Can you work these out from the model? Positions are in its coordinate system, mm. Give positions to 0.01 mm unless a question says otherwise; leave off trailing zeros. Order: outer loops, then holes, each group sorted by start corner. A loop starts at its lowest first (then second) coordinate and runs counter-clockwise, first axis right, second up. Notation, with made-up numbers: (15.25, 78.5) - (61.25, 78.5) arc R25 ccw to (61.25, 91.5) - close; hole circle Ø8 at (20.5, 28.5). An arc over 180 degrees is marked (long way). Answer as CSV lines item,"result".
```python
from build123d import *

# Parameters (mm, degrees)
CROQUIS1_W              = 762
CROQUIS1_H              = 76.2
SALIENTE_EXTRUIR1_DEPTH = 50.8
CROQUIS2_R              = 19.05
CORTAR_EXTRUIR5_DEPTH   = 387.255420674


with BuildPart() as part:
    # Croquis1 → Saliente-Extruir1 (new body)
    with BuildSketch(Plane.XY):
        Rectangle(CROQUIS1_W, CROQUIS1_H)
    extrude(amount=SALIENTE_EXTRUIR1_DEPTH)

    # Croquis2 → Cortar-Extruir5 (cut, through all)
    with BuildSketch(Plane(origin=(0, 0, 0), x_dir=(-1, 0, 0), z_dir=(0, 0, -1))):
        with Locations(Location((342.9, 0, 0), (0, 0, 180))):
            Circle(CROQUIS2_R)
    extrude(amount=-CORTAR_EXTRUIR5_DEPTH, mode=Mode.SUBTRACT)


solid = part.part
```
1) I want a section at C-C on z = 11.5. Write out the boundary of the cut face in (x, y), plus the area to 3 significant figures.
Answer block:
outline,"(-381, -38.1) - (381, -38.1) - (381, 38.1) - (-381, 38.1) - close; hole circle Ø38.1 at (-342.9, 0)"
area,"56,900 mm2"
2) I need wall thicknesses on line 1 along Y through (x, z) = (-342.9, 27.5); line 2 along X through (y, z) = (1.5, 22.5); line 3 along X through (y, z) = (11, 26.5). Which ranges of each line are inside material? Lowest first, please. Write a range as [from, to].
Answer block:
line 1,"[-38.1, -19.05], [19.05, 38.1]"
line 2,"[-381, -361.89], [-323.91, 381]"
line 3,"[-381, -358.45], [-327.35, 381]"
3) If we mould it in two halves opening along X, with no side actions, what happens to faces 1 (the flat face through (-381, -1, 25)), 2 (the cylindrical face through (-325.303, 7.296, 25.044)), 3 (the flat face through (-5, -38.1, 25))? For each: +X half, -X half, draft (parallel to the pull), parting line (faces both ways), or undercut.
Answer block:
face 1,"-X half"
face 2,"undercut"
face 3,"draft"
4) I want a section at B-B on y = 0. Write out the boundary of the cut face in (x, z), plus the area to 3 significant figures.
Answer block:
outline,"(-381, 0) - (-361.95, 0) - (-361.95, 50.8) - (-381, 50.8) - close; (-323.85, 0) - (381, 0) - (381, 50.8) - (-323.85, 50.8) - close"
area,"36,800 mm2"
5) I want a section at A-A on x = -342.9. Write out the boundary of the cut face in (y, z), plus the area to 3 significant figures.
Answer block:
outline,"(-38.1, 0) - (-19.05, 0) - (-19.05, 50.8) - (-38.1, 50.8) - close; (19.05, 0) - (38.1, 0) - (38.1, 50.8) - (19.05, 50.8) - close"
area,"1,940 mm2"
